```python
from build123d import *

# Parameters (mm, degrees)
BOSS_EXTRUDE1_DEPTH = 12.7


with BuildPart() as part:
    # Sketch1 → Boss-Extrude1 (new body)
    with BuildSketch(Plane(origin=(0, 0, 0), x_dir=(0, 0, -1), z_dir=(1, 0, 0))):
        Polygon((-160.02, -7.62), (-160.02, 69.196307345), (-121.92, 31.096307345), (-121.92, 69.196307345), (-83.82, 31.096307345), (-83.82, 69.196307345), (-45.72, 31.096307345), (-45.72, 69.196307345), (0, 23.476307345), (45.72, 69.196307345), (45.72, 31.096307345), (83.82, 69.196307345), (83.82, 31.096307345), (121.92, 69.196307345), (121.92, 31.096307345), (160.02, 69.196307345), (160.02, -7.62), align=None)
        Polygon((38.1, 12.7), (38.1, 50.8), (0, 12.7), (-38.1, 50.8), (-38.1, 12.7), (-76.2, 50.8), (-76.2, 12.7), (-114.3, 50.8), (-114.3, 12.7), (-152.4, 50.8), (-152.4, 0), (152.4, 0), (152.4, 50.8), (114.3, 12.7), (114.3, 50.8), (76.2, 12.7), (76.2, 50.8), align=None, mode=Mode.SUBTRACT)
    extrude(amount=BOSS_EXTRUDE1_DEPTH)


solid = part.part
```
For this review, take the finished solid that the model builds, in its own axes (mm). A direction names the side the tool comes from. Coordinates: 2 decimals unless noted, no trailing zeros. Write each loop counter-clockwise with the first axis right and the second up, starting at its lowest first coordinate (ties: lowest second). Pieces come first, ordered by that corner, then holes.
(1) Tool access review of faces 5 (the face through (6, -7.62, -2)), 6 (the face through (6.3, 31.5, 18.8)), 7 (the face through (6.261, 46.656, 23.18)): name each direction out of +Z, -Z, +X, -X, +Y, -Y from which nothing blocks a thin tool from reaching the whole face with its end or side.
(2) The part is to be moulded in two halves that separate along Y. For faces 1 (the face through (6, 0, 2)), 2 (the face through (6.261, 46.016, -22.54)), 3 (the face through (6, 32, 114.3)), 4 (the face through (6, 50, 83.82)), say which applies: +Y half, -Y half, draft (parallel to the pull), parting line (faces both ways), or undercut.
(3) Add section B-B on z = -128. Give the boundary of the cut face in (x, y).
(4) Wall thickness on probe 1 along Z at (x, y) = (10, 1); probe 2 along Y at (x, z) = (0.75, 44); probe 3 along Y at (x, z) = (10.75, -133): over which ranges is each line inside the solid? List them lowest first.
(5) For pin 1 Ø1 at (x, z) = (7.5, 115.5) entering from +Y; pin 2 Ø3 at (x, z) = (1.5, 17.5) entering from +Y, all flat-tipped, find the tip position at first contact; note any pin that passes through.
(6) Add section C-C on y = 58.5. Count the separate pieces of the cut face and the enclosed holes in it, then the cut area to 3 significant figures.
Answer sheet:
1. face 5: +Z, -Z, +X, -X, -Y
1. face 6: +X, -X
1. face 7: +X, -X, +Y
2. face 1: undercut
2. face 2: +Y half
2. face 3: undercut
2. face 4: draft
3. outline: (0, -7.62) - (12.7, -7.62) - (12.7, 0) - (0, 0) - close; (0, 26.4) - (12.7, 26.4) - (12.7, 37.18) - (0, 37.18) - close
4. probe 1: z = -160.02 to -152.4, 152.4 to 160.02
4. probe 2: y = -7.62 to 0, 18.6 to 67.48
4. probe 3: y = -7.62 to 0, 31.4 to 42.18
5. pin 1: stops at y = 63.28
5. pin 2: stops at y = 42.48
6. separate pieces: 8
6. enclosed holes: 0
6. area: 1,090 mm2
